```python
from build123d import *

# Parameters (mm, degrees)
SKETCH3_R                 = 20
BOSS_EXTRUDE2_DEPTH       = 3
BOSS_EXTRUDE3_DEPTH       = 3
CIRPATTERN1_COUNT         = 14
F_4_0MM_DOWEL_HOLE1_D     = 4
F_4_0MM_DOWEL_HOLE1_DEPTH = 3
F_4_0MM_DOWEL_HOLE1_TIP   = 1.201721238


with BuildPart() as part:
    # Sketch3 → Boss-Extrude2 (new body)
    with BuildSketch(Plane(origin=(0, 0, 0), x_dir=(0, 0, -1), z_dir=(1, 0, 0))):
        Circle(SKETCH3_R)
    extrude(amount=BOSS_EXTRUDE2_DEPTH)

    # Sketch4 → Boss-Extrude3 (add)
    with BuildSketch(Plane(origin=(3, 0, 0), x_dir=(0, 0, -1), z_dir=(1, 0, 0))):
        Polygon((1.5, 24.000314342), (2.617991667, 19.827912639), (-2.617991667, 19.827912639), (-1.5, 24.000314342), align=None)
    boss_extrude3 = extrude(amount=-BOSS_EXTRUDE3_DEPTH)

    # CirPattern1: Boss-Extrude3 ×14 about axis
    cirpattern1_axis = Axis((0, 0, 0), (1, 0, 0))
    for i in range(1, CIRPATTERN1_COUNT):
        add(boss_extrude3.rotate(cirpattern1_axis, i * 360 / CIRPATTERN1_COUNT))

    # Ø4.0mm Dowel Hole1
    with Locations(Plane(origin=(3, 0, 0), x_dir=(0, 0, -1), z_dir=(1, 0, 0))):
        with Locations((0, 0)):
            Hole(F_4_0MM_DOWEL_HOLE1_D / 2, depth=F_4_0MM_DOWEL_HOLE1_DEPTH)
            with Locations((0, 0, -(F_4_0MM_DOWEL_HOLE1_DEPTH + F_4_0MM_DOWEL_HOLE1_TIP / 2))):  # 118° drill point
                Cone(0, F_4_0MM_DOWEL_HOLE1_D / 2, F_4_0MM_DOWEL_HOLE1_TIP, mode=Mode.SUBTRACT)


solid = part.part
```
The listing builds one solid part. Answer for the finished solid, in the listing's coordinates (mm). A direction names the side the tool comes from. Round coordinates to 2 decimals unless told otherwise and drop trailing zeros. Write each loop counter-clockwise with the first axis right and the second up, starting at its lowest first coordinate (ties: lowest second). Pieces come first, ordered by that corner, then holes. Notation, with made-up numbers: (87.25, 52) -> (128.25, 52) arc R19 ccw to (128.25, 85) -> close; hole circle Ø2 at (89.5, 20). An arc over 180 degrees is marked (long way). Answer as a JSON object with one key per item and string values. Group by question number.
Q1. This flat-tipped pin is pushed along its axis until it touches: pin 1 Ø1 at (y, z) = (-16.5, 6) entering from -X. Where does it stop, or does it pass through?
Q2. Which of the six approach directions +Z, -Z, +X, -X, +Y, -Y give full straight-line access (tool end or side, diameter ignored) to faces 1 (the face through (1.521, 6.883, 20.937)), 2 (the face through (1.52, -15.26, 15.82)), 3 (the face through (1.521, -2.855, -21.796))?
Q3. Section B-B (y = 0) is taken. Write down the section's boundary in (x, z), plus the area to 3 significant figures.
Q4. Section A-A (z = 0) is taken. Write down the section's boundary in (x, y).
Q5. Determine the mould class of faces 4 (the face through (3, -5, 2)), 5 (the face through (1.521, 18.821, 11.358)), 6 (the face through (1.521, 15.285, 15.877)) for opening direction Z: pulls with the +Z half, pulls with the -Z half, needs draft (parallel to the pull), parting line crosses it, or undercut.
Q6. Straight lines are drawn through the part: line 1 along Z through (x, y) = (1.9, 0); line 2 along Y through (x, z) = (1, 18); line 3 along Y through (x, z) = (0.7, 0). For each, find the intervals that lie inside material, in ascending order.
Q7. Section C-C (y = -9) is taken. Write down the section's boundary in (x, z).
Check values:
{
 "1": {"pin 1": "x = 0"},
 "2": {"face 1": "+Z, +X, -X", "face 2": "+X, -X, -Y", "face 3": "-Z, +X, -X"},
 "3": {"outline": "(0, -20) -> (3, -20) -> (3, -2) -> (0, -2) -> close; (0, 2) -> (3, 2) -> (3, 20) -> (0, 20) -> close", "area": "108 mm^2"},
 "4": {"outline": "(0, -24) -> (3, -24) -> (3, -2) -> (0, -2) -> close; (0, 2) -> (3, 2) -> (3, 24) -> (0, 24) -> close"},
 "5": {"face 4": "needs draft", "face 5": "pulls with the +Z half", "face 6": "undercut"},
 "6": {"line 1": "-20 to -2, 2 to 20", "line 2": "-15.92 to -11.49, -8.72 to 8.72, 11.49 to 15.92", "line 3": "-24 to -2, 2 to 24"},
 "7": {"outline": "(0, -17.86) -> (3, -17.86) -> (3, 17.86) -> (0, 17.86) -> close"}
}
